```python
from build123d import *

# Parameters (mm, degrees)
CROQUIS3_W                                           = 42
CROQUIS3_H                                           = 42
SALIENTE_EXTRUIR1_DEPTH                              = 19.6
CROQUIS4_W                                           = 22.3
CROQUIS4_H                                           = 42
CROQUIS4_W_2                                         = 14.2
CROQUIS4_H_2                                         = 7.8
CORTAR_EXTRUIR1_DEPTH                                = 11.7
CROQUIS5_W                                           = 16.3
CROQUIS5_H                                           = 6.8
CROQUIS5_H_2                                         = 27.4
CORTAR_EXTRUIR2_DEPTH                                = 0.5
CORTAR_EXTRUIR3_START                                = -3.4
CORTAR_EXTRUIR3_DEPTH                                = 15.6
CROQUIS7_R                                           = 18.25
CORTAR_EXTRUIR4_DEPTH                                = 4
CROQUIS8_R                                           = 11.5
CORTAR_EXTRUIR5_DEPTH                                = 2
CROQUIS9_R                                           = 2.2
CORTAR_EXTRUIR6_DEPTH                                = 15.6
AVELLANADO_PARA_TORNILLO_CON_CABEZA_PLAN_D           = 3.4
AVELLANADO_PARA_TORNILLO_CON_CABEZA_PLAN_CSINK_D     = 6.3
AVELLANADO_PARA_TORNILLO_CON_CABEZA_PLAN_CSINK_ANGLE = 90
SALIENTE_EXTRUIR3_DEPTH                              = 1.9
CROQUIS13_R                                          = 8
CORTAR_EXTRUIR7_DEPTH                                = 0.5
CROQUIS14_R                                          = 5
CORTAR_EXTRUIR8_DEPTH                                = 2
DI_METRO_DE_TALADRO_7_6_7_6_1_D                      = 7.6
CROQUIS17_R                                          = 8
CORTAR_EXTRUIR9_DEPTH                                = 0.5
CROQUIS18_R                                          = 5
CORTAR_EXTRUIR10_DEPTH                               = 2
CROQUIS19_R                                          = 2.7
CORTAR_EXTRUIR11_DEPTH                               = 4.9
DI_METRO_DE_TALADRO_6_4_6_4_1_D                      = 6.4
DI_METRO_DE_TALADRO_6_4_6_4_1_DEPTH                  = 9.85
DI_METRO_DE_TALADRO_6_4_6_4_2_D                      = 6.4
DI_METRO_DE_TALADRO_6_4_6_4_2_DEPTH                  = 9.85


with BuildPart() as part:
    # Croquis3 → Saliente-Extruir1 (new body)
    with BuildSketch(Plane(origin=(0, 0, 0), x_dir=(1, 0, 0), z_dir=(0, 1, 0))):
        Rectangle(CROQUIS3_W, CROQUIS3_H)
    extrude(amount=-SALIENTE_EXTRUIR1_DEPTH)

    # Croquis4 → Cortar-Extruir1 (cut)
    with BuildSketch(Plane(origin=(0, 0, 0), x_dir=(1, 0, 0), z_dir=(0, 1, 0))):
        Rectangle(CROQUIS4_W, CROQUIS4_H)
        with Locations((0, 10.3)):
            Rectangle(CROQUIS4_W_2, CROQUIS4_H_2, mode=Mode.SUBTRACT)
    extrude(amount=-CORTAR_EXTRUIR1_DEPTH, mode=Mode.SUBTRACT)

    # Croquis5 → Cortar-Extruir2 (cut)
    with BuildSketch(Plane(origin=(0, -11.7, 0), x_dir=(1, 0, 0), z_dir=(0, 1, 0))):
        with Locations((0, 17.6)):
            Rectangle(CROQUIS5_W, CROQUIS5_H)
        with Locations((0, -7.3)):
            Rectangle(CROQUIS5_W, CROQUIS5_H_2)
    extrude(amount=-CORTAR_EXTRUIR2_DEPTH, mode=Mode.SUBTRACT)

    # Croquis6 → Cortar-Extruir3 (cut)
    with BuildSketch(Plane(origin=(0, -12.2, 0), x_dir=(1, 0, 0), z_dir=(0, 1, 0)).offset(CORTAR_EXTRUIR3_START)):
        with BuildLine():
            Line((4.1, -21), (4.1, -6.280127387))
            ThreePointArc((4.1, -6.280127387), (0, 7.5), (-4.1, -6.280127387))
            Line((-4.1, -6.280127387), (-4.1, -21))
            Line((-4.1, -21), (4.1, -21))
        make_face()
    extrude(amount=CORTAR_EXTRUIR3_DEPTH, mode=Mode.SUBTRACT)

    # Croquis7 → Cortar-Extruir4 (cut)
    with BuildSketch(Plane.XZ.offset(19.6)):
        Circle(CROQUIS7_R)
    extrude(amount=-CORTAR_EXTRUIR4_DEPTH, mode=Mode.SUBTRACT)

    # Croquis8 → Cortar-Extruir5 (cut)
    with BuildSketch(Plane.XZ.offset(15.6)):
        Circle(CROQUIS8_R)
    extrude(amount=-CORTAR_EXTRUIR5_DEPTH, mode=Mode.SUBTRACT)

    # Croquis9 → Cortar-Extruir6 (cut)
    with BuildSketch(Plane.XZ.offset(15.6)):
        with Locations((-16, 0)):
            Circle(CROQUIS9_R)
        with Locations((16, 0)):
            Circle(CROQUIS9_R)
    extrude(amount=-CORTAR_EXTRUIR6_DEPTH, mode=Mode.SUBTRACT)

    # Avellanado para tornillo con cabeza plana avellanada de M31 (through all)
    with Locations(Plane(origin=(0, 0, 0), x_dir=(1, 0, 0), z_dir=(0, 1, 0))):
        with Locations((-15.5, 15.5), (15.5, 15.5), (15.5, -15.5), (-15.5, -15.5)):
            CounterSinkHole(AVELLANADO_PARA_TORNILLO_CON_CABEZA_PLAN_D / 2, AVELLANADO_PARA_TORNILLO_CON_CABEZA_PLAN_CSINK_D / 2, counter_sink_angle=AVELLANADO_PARA_TORNILLO_CON_CABEZA_PLAN_CSINK_ANGLE)

    # Croquis12 → Saliente-Extruir3 (add)
    with BuildSketch(Plane(origin=(0, 0, 0), x_dir=(1, 0, 0), z_dir=(0, 1, 0))):
        with BuildLine():
            Line((-5.5, 12.7), (5.5, 12.7))
            ThreePointArc((5.5, 12.7), (7, 11.2), (5.5, 9.7))
            Line((5.5, 9.7), (-5.5, 9.7))
            ThreePointArc((-5.5, 9.7), (-7, 11.2), (-5.5, 12.7))
        make_face()
    extrude(amount=SALIENTE_EXTRUIR3_DEPTH)

    # Croquis13 → Cortar-Extruir7 (cut)
    with BuildSketch(Plane(origin=(21, 0, 0), x_dir=(0, 0, -1), z_dir=(1, 0, 0))):
        with Locations((-7.35, -6.3)):
            Circle(CROQUIS13_R)
    extrude(amount=-CORTAR_EXTRUIR7_DEPTH, mode=Mode.SUBTRACT)

    # Croquis14 → Cortar-Extruir8 (cut)
    with BuildSketch(Plane(origin=(20.5, 0, 0), x_dir=(0, 0, -1), z_dir=(1, 0, 0))):
        with Locations((-7.35, -6.3)):
            Circle(CROQUIS14_R)
    extrude(amount=-CORTAR_EXTRUIR8_DEPTH, mode=Mode.SUBTRACT)

    # Diámetro de taladro Ø7.6 (7.6)1 (through all)
    with Locations(Plane(origin=(18.5, 0, 0), x_dir=(0, 0, -1), z_dir=(1, 0, 0))):
        with Locations((-7.35, -6.3)):
            Hole(DI_METRO_DE_TALADRO_7_6_7_6_1_D / 2)

    # Croquis17 → Cortar-Extruir9 (cut)
    with BuildSketch(Plane.ZY.offset(21)):
        with Locations((7.35, -6.3)):
            Circle(CROQUIS17_R)
    extrude(amount=-CORTAR_EXTRUIR9_DEPTH, mode=Mode.SUBTRACT)

    # Croquis18 → Cortar-Extruir10 (cut)
    with BuildSketch(Plane.ZY.offset(20.5)):
        with Locations((7.35, -6.3)):
            Circle(CROQUIS18_R)
    extrude(amount=-CORTAR_EXTRUIR10_DEPTH, mode=Mode.SUBTRACT)

    # Croquis19 → Cortar-Extruir11 (cut)
    with BuildSketch(Plane(origin=(0, 0, -14.2), x_dir=(-1, 0, 0), z_dir=(0, 0, -1))):
        with Locations((4, -6.2)):
            Circle(CROQUIS19_R)
        with Locations((-4, -6.2)):
            Circle(CROQUIS19_R)
    extrude(amount=-CORTAR_EXTRUIR11_DEPTH, mode=Mode.SUBTRACT)

    # Diámetro de taladro Ø6.4 (6.4)1
    with Locations(Plane.ZY.offset(21)):
        with Locations((-7.6, -6.3)):
            Hole(DI_METRO_DE_TALADRO_6_4_6_4_1_D / 2, depth=DI_METRO_DE_TALADRO_6_4_6_4_1_DEPTH)

    # Diámetro de taladro Ø6.4 (6.4)2
    with Locations(Plane(origin=(21, 0, 0), x_dir=(0, 0, -1), z_dir=(1, 0, 0))):
        with Locations((7.6, -6.3)):
            Hole(DI_METRO_DE_TALADRO_6_4_6_4_2_D / 2, depth=DI_METRO_DE_TALADRO_6_4_6_4_2_DEPTH)


solid = part.part
```
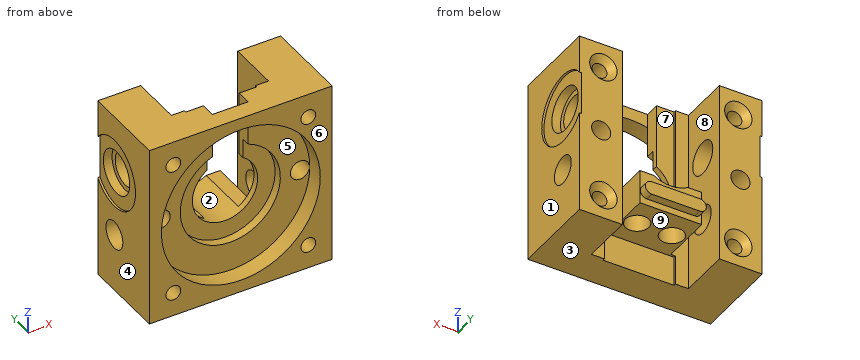
Verification items for the finished model (mm, model axes). Face numbers are marked on the shaded views. A direction names the side the tool comes from. Coordinates: 2 decimals unless noted, no trailing zeros. Write each loop counter-clockwise with the first axis right and the second up, starting at its lowest first coordinate (ties: lowest second). Pieces come first, ordered by that corner, then holes. Notation, with made-up numbers: (78.5, 88.5) - (116.5, 88.5) arc R25 ccw to (116.5, 119.5) - close; hole circle Ø3 at (-15.5, 26.25). An arc over 180 degrees is marked (long way). One line per question, with ' | ' between items. Start each with the question number.
1. Section check C-C (x = 15.5). Enter the section's corners in (y, z).
2. Section check B-B (y = -18). Enter the section's corners in (x, z).
3. Section check A-A (x = 0). Enter the section's corners in (y, z).
4. Section check D-D (z = -15.5). Enter the section's corners in (x, y), plus the area to 3 significant figures.
5. Material ranges on line 1 along X through (y, z) = (-5.5, -15.5); line 2 along Y through (x, z) = (-4, -10.95); line 3 along X through (y, z) = (-11.75, 16.5), recorded low to high.
6. Access from +Z, -Z, +X, -X, +Y, -Y to the whole of each face (thin tool, end or side, straight path). Record for the marked faces 5, 6, 7, 8 and 9.
7. Draft check along X on the marked faces 1, 2, 3 and 4. Enter one of: released by +X, released by -X, zero draft, split by the parting line, or undercut.
8. Gauge pin test, flat ends, axial feed: P1, Ø5, axis at x = -12, z = -13.5, coming from the +Y side; P2, Ø5, axis at x = -7, y = -6.5, coming from the -Z side; P3, Ø4, axis at x = 6.5, z = 5.5, coming from the +Y side. Record the tip position at first contact, or that the pin passes through.
Computed values:
1) outline: (-19.6, -21) - (0, -21) - (0, -18.65) - (-1.45, -17.2) - (-19.6, -17.2) - close; (-19.6, -13.8) - (-1.45, -13.8) - (0, -12.35) - (0, -2.14) - (-15.6, -2.14) - (-15.6, -9.63) - (-19.6, -9.63) - close; (-19.6, 9.63) - (-15.6, 9.63) - (-15.6, 2.14) - (0, 2.14) - (0, 12.35) - (-1.45, 13.8) - (-19.6, 13.8) - close; (-19.6, 17.2) - (-1.45, 17.2) - (0, 18.65) - (0, 21) - (-19.6, 21) - close; hole circle Ø7.6 at (-6.3, 7.35); hole circle Ø6.4 at (-6.3, -7.6)
2) outline: (-21, -21) - (21, -21) - (21, 21) - (-21, 21) - close; hole circle Ø36.5 at (0, 0); hole circle Ø3.4 at (-15.5, -15.5); hole circle Ø3.4 at (-15.5, 15.5); hole circle Ø3.4 at (15.5, -15.5); hole circle Ø3.4 at (15.5, 15.5)
3) outline: (-19.6, -21) - (-12.2, -21) - (-12.2, -14.2) - (0, -14.2) - (0, -12.7) - (1.9, -12.7) - (1.9, -9.7) - (0, -9.7) - (0, -7.5) - (-13.6, -7.5) - (-13.6, -11.5) - (-15.6, -11.5) - (-15.6, -18.25) - (-19.6, -18.25) - close; (-19.6, 18.25) - (-15.6, 18.25) - (-15.6, 21) - (-19.6, 21) - close
4) outline: (-21, -19.6) - (-17.2, -19.6) - (-17.2, -1.45) - (-18.65, 0) - (-21, 0) - close; (-13.8, -19.6) - (-9.63, -19.6) - (-9.63, -15.6) - (9.63, -15.6) - (9.63, -19.6) - (13.8, -19.6) - (13.8, -1.45) - (12.35, 0) - (11.15, 0) - (11.15, -11.7) - (8.15, -11.7) - (8.15, -12.2) - (-8.15, -12.2) - (-8.15, -11.7) - (-11.15, -11.7) - (-11.15, 0) - (-12.35, 0) - (-13.8, -1.45) - close; (17.2, -19.6) - (21, -19.6) - (21, 0) - (18.65, 0) - (17.2, -1.45) - close | area: 340 mm²
5) line 1: -21 to -17.2, -13.8 to -11.15, 11.15 to 13.8, 17.2 to 21 | line 2: -15.6 to -8.9, -3.5 to 1.9 | line 3: -21 to -16.87, -14.13 to -8.15, 8.15 to 14.13, 16.87 to 21
6) face 5: -Y | face 6: +Z, -Z, +X, -X, -Y | face 7: +Z, +Y | face 8: +Z, -Z, +Y | face 9: -Z, +Y
7) face 1: released by +X | face 2: undercut | face 3: zero draft | face 4: released by -X
8) P1: y = 0 | P2: z = -14.2 | P3: y = -11.7
